Input: part model. Units: mm. Frame: model coordinates. A direction names the side the tool comes from. Round coordinates to 2 decimals unless told otherwise and drop trailing zeros. Loops run counter-clockwise (first coordinate to the right, second up) from the corner with the lowest first, then second, coordinate; pieces in that order, holes last. Notation, with made-up numbers: M -2.5,89.25 L 18.5,89.25 A22 cw 18.5,124.25 Z; hole C 27,-37.5 d10. An arc over 180 degrees is marked long. Put each result on its own line as item: value. Start each with the question number.
1) Line query: probe 1 along Y at (x, z) = (-139.7, 129.5); probe 2 along Z at (x, y) = (-62, 12) (3 decimals); probe 3 along Y at (x, z) = (-90, 122) (3 decimals). Output: solid intervals per line, ascending.
2) Section D-D on z = 112.5. Output: boundary loops of the cut face in (x, y) (3 decimals).
3) Section B-B on x = 99.5. Output: boundary loops of the cut face in (y, z) (3 decimals), plus the area to 3 significant figures.
4) Section C-C on z = 123.5. Output: boundary loops of the cut face in (x, y) (3 decimals).
5) Reachability of faces 1 (the face through (2, 3.175, 116)), 2 (the face through (144.344, 2.293, 122.119)) from +Z, -Z, +X, -X, +Y, -Y: full face, straight path, thin tool, end or side. Return the list, or none.
6) Section A-A on x = -139.7. Output: boundary loops of the cut face in (y, z) (3 decimals), plus the area to 3 significant figures.
7) Pin query (flat end, axial travel): pin 1 (10 mm diameter, centred on y = 11, z = 122.5, fed in from +X) (3 decimals); pin 2 (10 mm diameter, centred on x = 91, y = 14.5, fed in from -Z); pin 3 (3 mm diameter, centred on x = 120, z = 124, fed in from +Y) (3 decimals). Return the tip coordinate at first contact, or that it passes through.
8) Draft query along X for faces 3 (the face through (-143.665, 12.874, 128.61)), 4 (the face through (-144.344, 2.293, 122.119)), 5 (the face through (-51.704, 10.24, 128.61)), 6 (the face through (2, 13, 130.175)). Return one class per face: +X half, -X half, draft (parallel to the pull), parting line (faces both ways), or undercut.
from build123d import *

# Parameters (mm, degrees)
PAD6966_DEPTH   = 152.4
POCKET672_DEPTH = 25.401
SKETCH7924_R    = 2.38125
SKETCH7924_R_2  = 3.96875
POCKET673_DEPTH = 25.401


with BuildPart() as part:
    # Sketch7922 → Pad6966 (new body, symmetric)
    with BuildSketch(Plane.YZ):
        Polygon((0, 0), (0, -25.4), (3.175, -25.4), (3.175, -3.175), (25.4, -3.175), (25.4, 0), align=None)
    extrude(amount=PAD6966_DEPTH, both=True)

    # Sketch7923 → Pocket672 (cut, through all)
    with BuildSketch(Plane.XZ):
        Polygon((-114.3, -38.1), (-152.4, 0), (-152.4, -38.1), align=None)
        Polygon((114.3, -38.1), (152.4, 0), (152.4, -38.1), align=None)
    extrude(amount=-POCKET672_DEPTH, mode=Mode.SUBTRACT)

    # Sketch7924 → Pocket673 (cut, through all)
    with BuildSketch(Plane.XY):
        with Locations((-53.975, 9.525)):
            Circle(SKETCH7924_R)
        with Locations((53.975, 9.525)):
            Circle(SKETCH7924_R)
        with Locations((-139.7, 12.7)):
            Circle(SKETCH7924_R_2)
    extrude(amount=-POCKET673_DEPTH, mode=Mode.SUBTRACT)


with BuildPart() as part_1:
    # Body6272 placement: moved
    add(part.part.moved(Location((0, 0, 130.175))))


solid = part_1.part
Geometry results:
1. probe 1: y = 0 to 8.73, 16.67 to 25.4
1. probe 2: z = 127 to 130.175
1. probe 3: y = 0 to 3.175
2. outline: M -134.725,0 L 134.725,0 L 134.725,3.175 L -134.725,3.175 Z
3. outline: M 0,104.775 L 3.175,104.775 L 3.175,127 L 25.4,127 L 25.4,130.175 L 0,130.175 Z
3. area: 151 mm²
4. outline: M -145.725,0 L 145.725,0 L 145.725,3.175 L -145.725,3.175 Z
5. face 1: -Z, +X, -X, +Y
5. face 2: -Z, +X, +Y, -Y
6. outline: M 0,117.475 L 3.175,117.475 L 3.175,127 L 8.731,127 L 8.731,130.175 L 0,130.175 Z; M 16.669,127 L 25.4,127 L 25.4,130.175 L 16.669,130.175 Z
6. area: 85.7 mm²
7. pin 1: stops at x = 149.725
7. pin 2: stops at z = 127
7. pin 3: stops at y = 3.175
8. face 3: undercut
8. face 4: -X half
8. face 5: undercut
8. face 6: draft
